Build history of the part. All positions in model axes, mm. Face numbers are marked on the shaded views. A direction names the side the tool comes from. Give positions to 0.01 mm unless a question says otherwise; leave off trailing zeros. Order: outer loops, then holes, each group sorted by start corner. A loop starts at its lowest first (then second) coordinate and runs counter-clockwise, first axis right, second up. Notation, with made-up numbers: (42, 13) - (64, 13) arc R28 ccw to (64, 32) - close; hole circle Ø5 at (-17, 77.25). An arc over 180 degrees is marked (long way). Answer in a Markdown table with one row per item.
```python
from build123d import *

# Parameters (mm, degrees)
ESBO_O1_R                = 29.6
RESSALTO_EXTRUS_O1_DEPTH = 8
CORTE_EXTRUS_O2_DEPTH    = 8
ESBO_O4_R                = 1.5
CORTE_EXTRUS_O4_DEPTH    = 8


with BuildPart() as part:
    # Esboço1 → Ressalto-extrusão1 (new body)
    with BuildSketch(Plane(origin=(0, 0, 0), x_dir=(1, 0, 0), z_dir=(0, 1, 0))):
        with Locations(Location((-36.441507633, 11.937959287, 0), (0, 0, 270))):
            Circle(ESBO_O1_R)
    extrude(amount=RESSALTO_EXTRUS_O1_DEPTH)

    # Esboço2 → Corte-extrusão2 (cut)
    with BuildSketch(Plane(origin=(0, 8, 0), x_dir=(1, 0, 0), z_dir=(0, 1, 0))):
        with BuildLine():
            ThreePointArc((-46.052507633, 11.937959287), (-45.32091382, 15.615929755), (-43.237510907, 18.733962561))
            Line((-43.237510907, 18.733962561), (-50.583643257, 26.080094911))
            ThreePointArc((-50.583643257, 26.080094911), (-54.919098283, 19.591627934), (-56.441507633, 11.937959287))
            Line((-56.441507633, 11.937959287), (-46.052507633, 11.937959287))
        make_face()
        with BuildLine():
            ThreePointArc((-36.441507633, 21.548959287), (-32.763537165, 20.817365474), (-29.645504359, 18.733962561))
            Line((-29.645504359, 18.733962561), (-22.299372009, 26.080094911))
            ThreePointArc((-22.299372009, 26.080094911), (-28.787838986, 30.415549937), (-36.441507633, 31.937959287))
            Line((-36.441507633, 31.937959287), (-36.441507633, 21.548959287))
        make_face()
        with BuildLine():
            Line((-16.441507633, 11.937959287), (-26.830507633, 11.937959287))
            ThreePointArc((-26.830507633, 11.937959287), (-27.562101446, 8.259988818), (-29.645504359, 5.141956013))
            Line((-29.645504359, 5.141956013), (-22.299372009, -2.204176337))
            ThreePointArc((-22.299372009, -2.204176337), (-17.963916983, 4.28429064), (-16.441507633, 11.937959287))
        make_face()
        with BuildLine():
            Line((-36.441507633, -8.062040713), (-36.441507633, 2.326959287))
            ThreePointArc((-36.441507633, 2.326959287), (-40.119478102, 3.0585531), (-43.237510907, 5.141956013))
            Line((-43.237510907, 5.141956013), (-50.583643257, -2.204176337))
            ThreePointArc((-50.583643257, -2.204176337), (-44.09517628, -6.539631363), (-36.441507633, -8.062040713))
        make_face()
    extrude(amount=-CORTE_EXTRUS_O2_DEPTH, mode=Mode.SUBTRACT)

    # Esboço4 → Corte-extrusão4 (cut)
    with BuildSketch(Plane(origin=(0, 8, 0), x_dir=(1, 0, 0), z_dir=(0, 1, 0))):
        with Locations(Location((-30.091507633, 11.937959287, 0), (0, 0, 270))):
            Circle(ESBO_O4_R)
        with Locations(Location((-42.791507633, 11.937959287, 0), (0, 0, 270))):
            Circle(ESBO_O4_R)
    extrude(amount=-CORTE_EXTRUS_O4_DEPTH, mode=Mode.SUBTRACT)


solid = part.part
```
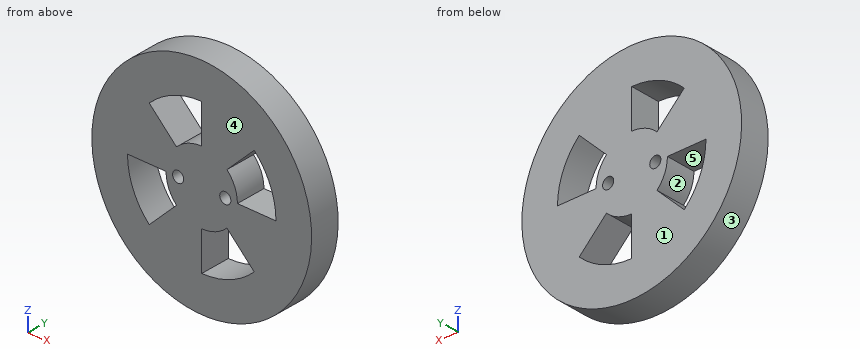
1. Two-plate mould, pull along Z, no slides. Class the marked faces 3, 4 and 5: +Z half, -Z half, draft (parallel to the pull), parting line (faces both ways), or undercut.
Check result:
| item | result |
|---|---|
| face 3 | parting line |
| face 4 | draft |
| face 5 | undercut |
2. Which spindle directions (+Z, -Z, +X, -X, +Y, -Y) get a long thin tool onto all of the face, cutting with end or side? Do the marked faces 1 and 2. Say none if no direction does.
Check result:
| item | result |
|---|---|
| face 1 | +Z, -Z, +X, -X, +Y |
| face 2 | +Y, -Y |
3. Cut at B-B on x = -19. Write the cut outline in (y, z).
Check result:
| item | result |
|---|---|
| outline | (0, -35.85) - (8, -35.85) - (8, -11.94) - (0, -11.94) - close; (0, -2.15) - (8, -2.15) - (8, 11.98) - (0, 11.98) - close |
4. Cut at A-A on z = -4. Write the cut outline in (x, y).
Check result:
| item | result |
|---|---|
| outline | (-64.96, 0) - (-44.38, 0) - (-44.38, 8) - (-64.96, 8) - close; (-41.86, 0) - (-28.5, 0) - (-28.5, 8) - (-41.86, 8) - close; (-18.08, 0) - (-7.93, 0) - (-7.93, 8) - (-18.08, 8) - close |
5. Cut at C-C on y = 5.75. Write the cut outline in (x, z), and give its area (3 significant figures).
Check result:
| item | result |
|---|---|
| outline | circle Ø59.2 at (-36.44, -11.94); hole (-56.44, -11.94) arc R20 ccw to (-50.58, -26.08) - (-43.24, -18.73) arc R9.61 cw to (-46.05, -11.94) - close; hole (-50.58, 2.2) - (-43.24, -5.14) arc R9.61 cw to (-36.44, -2.33) - (-36.44, 8.06) arc R20 ccw to start; hole circle Ø3 at (-42.79, -11.94); hole (-36.44, -31.94) arc R20 ccw to (-22.3, -26.08) - (-29.65, -18.73) arc R9.61 cw to (-36.44, -21.55) - close; hole circle Ø3 at (-30.09, -11.94); hole (-29.65, -5.14) arc R9.61 cw to (-26.83, -11.94) - (-16.44, -11.94) arc R20 ccw to (-22.3, 2.2) - close |
| area | 2,260 mm² |
6. Cut at D-D on x = -52.5. Write the cut outline in (y, z).
Check result:
| item | result |
|---|---|
| outline | (0, -36.8) - (8, -36.8) - (8, -23.86) - (0, -23.86) - close; (0, -11.94) - (8, -11.94) - (8, 12.93) - (0, 12.93) - close |
7. Drop flat-ended pins along their axis: P1, Ø1.5, axis at x = -43.5, y = 4.5, coming from the +Z side; P2, Ø4, axis at y = 5.5, z = -27, coming from the +X side; P3, Ø2.5, axis at x = -30.09, z = -11.94, coming from the -Y side; P4, Ø2.5, axis at x = -24, y = 3.5, coming from the +Z side. Give the stop position or say it passes through.
Check result:
| item | result |
|---|---|
| P1 | stops at z = 16.98 |
| P2 | stops at x = -9.88 |
| P3 | passes through |
| P4 | stops at z = 15.46 |
8. Probe line 1 (X direction, y = 3.5, z = -25); line 2 (Z direction, x = -25, y = 5.25); line 3 (Z direction, x = -23.5, y = 7). List the from-to ranges inside material, lowest first.
Check result:
| item | result |
|---|---|
| line 1 | x = -63 to -51.59, -49.5 to -36.44, -23.38 to -9.88 |
| line 2 | z = -39.24 to -28.34, -23.38 to -11.94, -0.5 to 15.36 |
| line 3 | z = -38.56 to -27.19, -24.88 to -11.94, 1 to 14.68 |
